Here's how the part is built. I have some questions about the finished solid (model axes, mm). Face numbers are marked on the shaded views. A direction names the side the tool comes from. Round coordinates to 2 decimals unless told otherwise and drop trailing zeros. Write each loop counter-clockwise with the first axis right and the second up, starting at its lowest first coordinate (ties: lowest second). Pieces come first, ordered by that corner, then holes. Notation, with made-up numbers: (77, 39) -> (85, 39) arc R19 cw to (85, 71) -> close; hole circle Ø4 at (25.25, -25.75). An arc over 180 degrees is marked (long way). Answer in a Markdown table with one row per item.
from build123d import *

# Parameters (mm, degrees)
SKETCH1_W                 = 14
SKETCH1_H                 = 14
BOSS_EXTRUDE1_DEPTH       = 30
SKETCH2_R                 = 5.5
BOSS_EXTRUDE2_DEPTH       = 1.5
SKETCH3_R                 = 2
BOSS_EXTRUDE4_DEPTH       = 13.5
SKETCH7_R                 = 2
BOSS_EXTRUDE6_DEPTH       = 10
CHAMFER1_SIZE             = 0.5
M2X0_4_TAPPED_HOLE1_D     = 1.6
M2X0_4_TAPPED_HOLE1_DEPTH = 4.4
M2X0_4_TAPPED_HOLE1_TIP   = 0.480688495
FILLET1_R                 = 0.75
CHAMFER2_SIZE             = 0.25
M2X0_4_TAPPED_HOLE2_D     = 1.6
M2X0_4_TAPPED_HOLE2_DEPTH = 4.4
M2X0_4_TAPPED_HOLE2_TIP   = 0.480688495


with BuildPart() as part:
    # Sketch1 → Boss-Extrude1 (new body)
    with BuildSketch(Plane.XY):
        Rectangle(SKETCH1_W, SKETCH1_H)
    extrude(amount=BOSS_EXTRUDE1_DEPTH)

    # Sketch2 → Boss-Extrude2 (add)
    with BuildSketch(Plane(origin=(0, 0, 0), x_dir=(-1, 0, 0), z_dir=(0, 0, -1))):
        Circle(SKETCH2_R)
    extrude(amount=BOSS_EXTRUDE2_DEPTH)

    # Sketch3 → Boss-Extrude4 (add)
    with BuildSketch(Plane(origin=(0, 0, -1.5), x_dir=(-1, 0, 0), z_dir=(0, 0, -1))):
        Circle(SKETCH3_R)
    extrude(amount=BOSS_EXTRUDE4_DEPTH)

    # Sketch7 → Boss-Extrude6 (add)
    with BuildSketch(Plane.XY.offset(30)):
        Circle(SKETCH7_R)
    extrude(amount=BOSS_EXTRUDE6_DEPTH)

    # Chamfer1
    chamfer1_edges = [part.edges().sort_by_distance(p)[0] for p in [
        (2, 0, -15),
        (-2, 0, 40),
    ]]
    chamfer(chamfer1_edges, length=CHAMFER1_SIZE)

    # M2x0.4 Tapped Hole1
    with Locations(Plane(origin=(0, 0, 0), x_dir=(-1, 0, 0), z_dir=(0, 0, -1))):
        with Locations((5.75, 5.75), (-5.75, 5.75), (-5.75, -5.75), (5.75, -5.75)):
            Hole(M2X0_4_TAPPED_HOLE1_D / 2, depth=M2X0_4_TAPPED_HOLE1_DEPTH)
            with Locations((0, 0, -(M2X0_4_TAPPED_HOLE1_DEPTH + M2X0_4_TAPPED_HOLE1_TIP / 2))):  # 118° drill point
                Cone(0, M2X0_4_TAPPED_HOLE1_D / 2, M2X0_4_TAPPED_HOLE1_TIP, mode=Mode.SUBTRACT)

    # Fillet1
    fillet1_edges = [part.edges().sort_by_distance(p)[0] for p in [
        (7, -7, 15),
        (-7, -7, 15),
        (-7, 7, 15),
        (7, 7, 15),
    ]]
    fillet(fillet1_edges, radius=FILLET1_R)

    # Chamfer2
    chamfer2_edges = [part.edges().sort_by_distance(p)[0] for p in [
        (0, 7, 0),
        (0, 7, 30),
        (7, 0, 0),
        (0, -7, 0),
        (-7, 0, 0),
        (-6.780330086, 6.780330086, 0),
        (-6.780330086, -6.780330086, 0),
        (6.780330086, -6.780330086, 0),
        (6.780330086, 6.780330086, 0),
        (7, 0, 30),
        (-7, 0, 30),
        (0, -7, 30),
        (-6.780330086, 6.780330086, 30),
        (-6.780330086, -6.780330086, 30),
        (6.780330086, -6.780330086, 30),
        (6.780330086, 6.780330086, 30),
    ]]
    chamfer(chamfer2_edges, length=CHAMFER2_SIZE)

    # M2x0.4 Tapped Hole2
    with Locations(Plane.XY.offset(30)):
        with Locations((5.75, 5.75), (-5.75, -5.75)):
            Hole(M2X0_4_TAPPED_HOLE2_D / 2, depth=M2X0_4_TAPPED_HOLE2_DEPTH)
            with Locations((0, 0, -(M2X0_4_TAPPED_HOLE2_DEPTH + M2X0_4_TAPPED_HOLE2_TIP / 2))):  # 118° drill point
                Cone(0, M2X0_4_TAPPED_HOLE2_D / 2, M2X0_4_TAPPED_HOLE2_TIP, mode=Mode.SUBTRACT)


solid = part.part
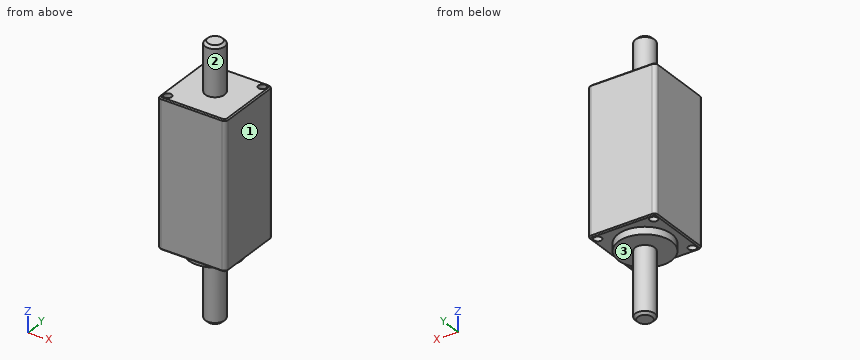
1) For pin 1 (1.3 mm diameter, centred on x = -5.75, y = -5.75, fed in from +Z); pin 2 (5 mm diameter, centred on x = -1.5, y = -5, fed in from -Z); pin 3 (1.5 mm diameter, centred on y = -1, z = -1.5, fed in from +X); pin 4 (5.5 mm diameter, centred on x = 0.5, y = 2, fed in from -Z), each with a flat end and sliding along its axis, tell me the tip position at first contact or that it passes through.
Response:
| item | result |
|---|---|
| pin 1 | stops at z = 25.51 |
| pin 2 | stops at z = -1.5 |
| pin 3 | stops at x = 5.49 |
| pin 4 | stops at z = -15 |
2) I need wall thicknesses on line 1 (Y direction, x = -5.75, z = 1.65); line 2 (Y direction, x = -5.75, z = 27.85). Which ranges of each line are inside material? Lowest first, please. Write a range as [from, to].
Response:
| item | result |
|---|---|
| line 1 | y = [-7, -6.55], [-4.95, 4.95], [6.55, 7] |
| line 2 | y = [-7, -6.55], [-4.95, 7] |
3) Which directions (+Z, -Z, +X, -X, +Y, -Y) give clear straight access to the entire face, cutting with the end or side of a thin tool? Please do the marked faces 1, 2 and 3.
Response:
| item | result |
|---|---|
| face 1 | +Z, -Z, +X, +Y, -Y |
| face 2 | +Z |
| face 3 | -Z |
4) I want a section at A-A, the plane y = 0. List the corners of the cut face in (x, z) for me, and give its area (3 significant figures).
Response:
| item | result |
|---|---|
| outline | (-7, 0.25) -> (-6.75, 0) -> (-5.5, 0) -> (-5.5, -1.5) -> (-2, -1.5) -> (-2, -14.5) -> (-1.5, -15) -> (1.5, -15) -> (2, -14.5) -> (2, -1.5) -> (5.5, -1.5) -> (5.5, 0) -> (6.75, 0) -> (7, 0.25) -> (7, 29.75) -> (6.75, 30) -> (2, 30) -> (2, 39.5) -> (1.5, 40) -> (-1.5, 40) -> (-2, 39.5) -> (-2, 30) -> (-6.75, 30) -> (-7, 29.75) -> close |
| area | 530 mm^2 |
5) I want a section at D-D, the plane x = 3.75. List the corners of the cut face in (y, z) for me.
Response:
| item | result |
|---|---|
| outline | (-7, 0.25) -> (-6.75, 0) -> (-4.02, 0) -> (-4.02, -1.5) -> (4.02, -1.5) -> (4.02, 0) -> (6.75, 0) -> (7, 0.25) -> (7, 29.75) -> (6.75, 30) -> (-6.75, 30) -> (-7, 29.75) -> close |
6) I want a section at C-C, the plane z = -9. List the corners of the cut face in (x, y) for me, and give its area (3 significant figures).
Response:
| item | result |
|---|---|
| outline | circle Ø4 at (0, 0) |
| area | 12.6 mm^2 |
